Here's the drawing with two shaded views (mm, measured from the low corner). I have some questions. Give positions to 0.01 mm unless a question says otherwise; leave off trailing zeros. Loops run counter-clockwise (first coordinate to the right, second up) from the corner with the lowest first, then second, coordinate; pieces in that order, holes last.
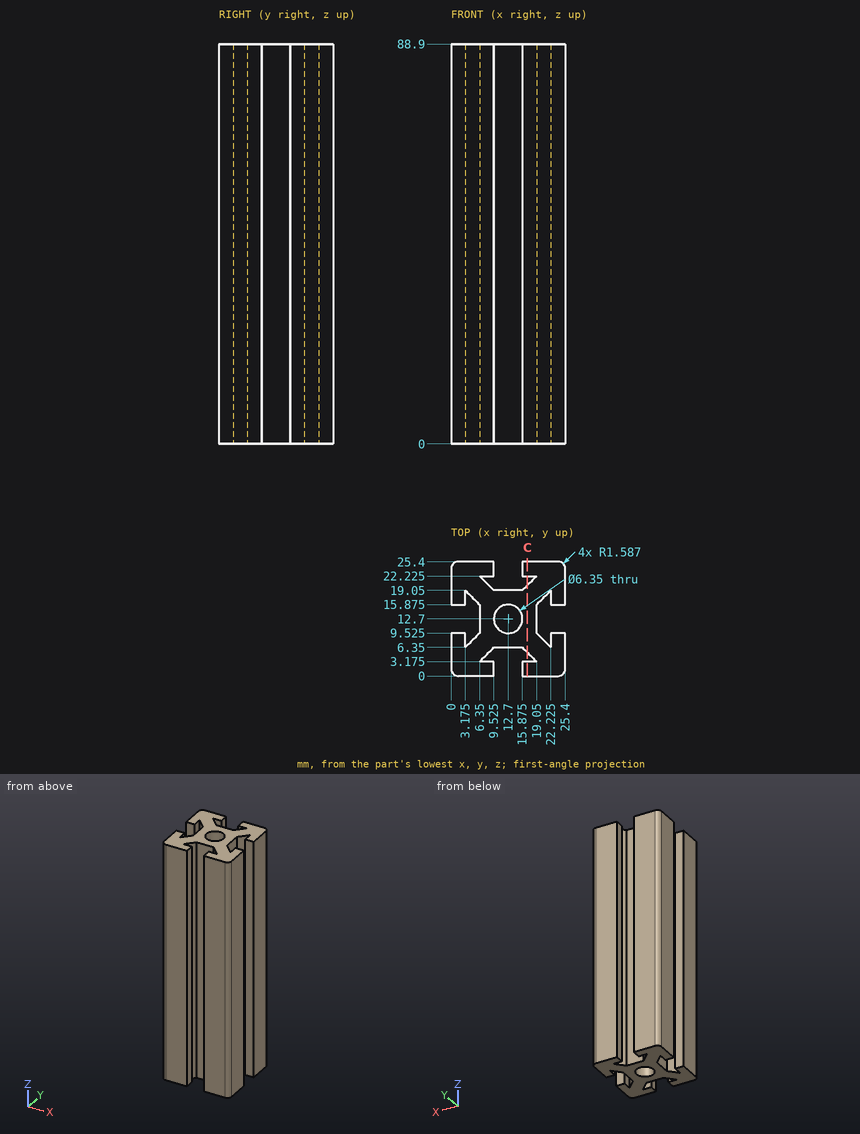
(1) Please list where these lines run through material, in increasing order: probe 1 along Y at (x, z) = (17, 83) (1 decimal); probe 2 along X at (y, z) = (7, 41.5) (1 decimal); probe 3 along Y at (x, z) = (8.5, 52) (1 decimal).
Returned:
probe 1: y = 0 to 3.2, 5.2 to 20.2, 22.2 to 25.4
probe 2: x = 0 to 3.2, 3.8 to 21.6, 22.2 to 25.4
probe 3: y = 0 to 3.2, 5.3 to 20.1, 22.2 to 25.4
(2) Will these pins go through, and if not, where does the flat tip stop? P1, Ø1, axis at y = 1, z = 42, coming from the -X side; P2, Ø1, axis at x = 13.5, z = 26.5, coming from the +Y side.
Returned:
P1: stops at x = 0
P2: stops at y = 19.05
(3) Suppose I cut it at C-C on x = 17. List the corners of the cut face in (y, z) for me (1 decimal).
Returned:
outline: (0, 0) - (3.2, 0) - (3.2, 88.9) - (0, 88.9) - close; (5.2, 0) - (20.2, 0) - (20.2, 88.9) - (5.2, 88.9) - close; (22.2, 0) - (25.4, 0) - (25.4, 88.9) - (22.2, 88.9) - close
